```python
from build123d import *

# Parameters (mm, degrees)
BOSS_EXTRUDE1_DEPTH = 2
BOSS_EXTRUDE2_START = -17.5
SKETCH2_R           = 1.75
BOSS_EXTRUDE2_DEPTH = 35
SKETCH3_R           = 3
CUT_EXTRUDE1_DEPTH  = 6.75
CUT_EXTRUDE2_DEPTH  = 2
BOSS_EXTRUDE4_START = -0.5
BOSS_EXTRUDE4_DEPTH = 3.5
SKETCH6_R           = 1.75
CUT_EXTRUDE3_DEPTH  = 77.941536247
FILLET1_R           = 1
SKETCH7_W           = 9
SKETCH7_H           = 6
CUT_EXTRUDE4_DEPTH  = 2
FILLET2_R           = 3
FILLET3_R           = 3


# Some blends are built 0.0001 mm under size
with BuildPart() as part:
    # Sketch1 → Boss-Extrude1 (new body)
    with BuildSketch(Plane(origin=(0, 0, 0), x_dir=(1, 0, 0), z_dir=(0, 1, 0))):
        with BuildLine():
            Line((-17.5, -42), (17.5, -42))
            ThreePointArc((17.5, -42), (45.5, 0), (17.5, 42))
            Line((17.5, 42), (-17.5, 42))
            ThreePointArc((-17.5, 42), (-45.5, 0), (-17.5, -42))
        make_face()
    extrude(amount=BOSS_EXTRUDE1_DEPTH)

    # Sketch2 → Boss-Extrude2 (add)
    with BuildSketch(Plane(origin=(0, 0, 0), x_dir=(0, 0, -1), z_dir=(1, 0, 0)).offset(BOSS_EXTRUDE2_START)):
        with BuildLine():
            Line((-42, 0), (-42.171572875, 0))
            ThreePointArc((-42.171572875, 0), (-48, 1), (-42.171572875, 2))
            Line((-42.171572875, 2), (-42, 2))
            Line((-42, 2), (-42, 1))
            Line((-42, 1), (-42, 0))
        make_face()
        with Locations((-45, 1)):
            Circle(SKETCH2_R, mode=Mode.SUBTRACT)
    extrude(amount=BOSS_EXTRUDE2_DEPTH)

    # Sketch3 → Cut-Extrude1 (cut)
    with BuildSketch(Plane(origin=(3.5, 0, 0), x_dir=(0, 0, -1), z_dir=(1, 0, 0))):
        with Locations((-45, 1)):
            Circle(SKETCH3_R)
    cut_extrude1 = extrude(amount=CUT_EXTRUDE1_DEPTH, mode=Mode.SUBTRACT)

    # Mirror1: Cut-Extrude1 across plane
    add(cut_extrude1.mirror(Plane(origin=(0, 0, 0), x_dir=(0, 0, 1), z_dir=(1, 0, 0))), mode=Mode.SUBTRACT)

    # Sketch4 → Cut-Extrude2 (cut)
    with BuildSketch(Plane(origin=(0, 2, 0), x_dir=(1, 0, 0), z_dir=(0, 1, 0))):
        Polygon((0.75, 42), (21.25, 42), (21.25, 32.75), (0.75, 32.75), (0.75, 35), (-17.5, 35), (-17.5, 42), align=None)
    extrude(amount=-CUT_EXTRUDE2_DEPTH, mode=Mode.SUBTRACT)

    # Sketch5 → Boss-Extrude4 (add)
    with BuildSketch(Plane(origin=(-17.5, 0, 0), x_dir=(0, 0, -1), z_dir=(1, 0, 0)).offset(BOSS_EXTRUDE4_START)):
        with BuildLine():
            Line((35, 1), (35, 2))
            Line((35, 2), (38.171572875, 2))
            ThreePointArc((38.171572875, 2), (44, 1), (38.171572875, 0))
            Line((38.171572875, 0), (35, 0))
            Line((35, 0), (35, 1))
        make_face()
    extrude(amount=BOSS_EXTRUDE4_DEPTH)

    # Sketch6 → Cut-Extrude3 (cut, through all)
    with BuildSketch(Plane(origin=(-14.5, 0, 0), x_dir=(0, 0, -1), z_dir=(1, 0, 0))):
        with Locations((41, 1)):
            Circle(SKETCH6_R)
    extrude(amount=-CUT_EXTRUDE3_DEPTH, mode=Mode.SUBTRACT)

    # Fillet1
    fillet1_edges = [part.edges().sort_by_distance(p)[0] for p in [
        (-20.235557777, 0, -39.563859338),
        (-20.235557777, 2, -39.563859338),
    ]]
    fillet(fillet1_edges, radius=FILLET1_R - 0.0001)  # a hair under: the kernel refuses the full size

    # Sketch7 → Cut-Extrude4 (cut)
    with BuildSketch(Plane(origin=(0, 2, 0), x_dir=(1, 0, 0), z_dir=(0, 1, 0))):
        with Locations((24.75, 38)):
            Rectangle(SKETCH7_W, SKETCH7_H)
    extrude(amount=-CUT_EXTRUDE4_DEPTH, mode=Mode.SUBTRACT)

    # Fillet2
    # the kernel refuses this fillet: 3 mm, written as the material it adds along each edge
    with BuildSketch(Plane(origin=(-14.5, 0, -35), x_dir=(0, 0, -1), z_dir=(0, 1, 0))) as fillet2_piece_1:
        with BuildLine():
            CenterArc((FILLET2_R, -FILLET2_R), FILLET2_R, 90, 90)
            Line((0, -FILLET2_R), (0, 0))
            Line((0, 0), (FILLET2_R, 0))
        make_face()
    extrude(amount=2)
    # the kernel refuses this fillet: 3 mm, written as the material it takes off along each edge
    with BuildSketch(Plane(origin=(29.07318352, 4.856917414, -35), x_dir=(-1, 0, 0), z_dir=(0, -1, 0))) as fillet2_2_piece_1:
        with BuildLine():
            CenterArc((1.104450978, -3), FILLET2_R, 90, 41.15420196)
            ThreePointArc((-0.869812495, -0.741176471), (-0.43723324, -0.367857378), (0, 0))
            Line((0, 0), (1.104450978, 0))
        make_face()
    extrude(amount=7.713834827, mode=Mode.SUBTRACT)
    with BuildSketch(Plane(origin=(21.25, -7.261843774, -35), x_dir=(0, 0, 1), z_dir=(0, 1, 0))) as fillet2_2_piece_2:
        with BuildLine():
            CenterArc((3, 2.90473751), FILLET2_R, 180, 75.522487814)
            Line((0, 2.90473751), (0, 0))
            Line((0, 0), (2.25, 0))
        make_face()
    extrude(amount=16.523687548, mode=Mode.SUBTRACT)
    with BuildSketch(Plane(origin=(0.75, 9.261843774, -35), x_dir=(-1, 0, 0), z_dir=(0, -1, 0))) as fillet2_2_piece_3:
        with BuildLine():
            CenterArc((2.90473751, -3), FILLET2_R, 90, 75.522487814)
            Line((0, -2.25), (0, 0))
            Line((0, 0), (2.90473751, 0))
        make_face()
    extrude(amount=16.523687548, mode=Mode.SUBTRACT)

    # Fillet3
    fillet3_edges = [part.edges().sort_by_distance(p)[0] for p in [
        (21.25, 1, -32.75),
        (0.75, 1, -32.75),
    ]]
    fillet(fillet3_edges, radius=FILLET3_R)


solid = part.part
```
Geometry: final body of the model. Coordinates: model frame, mm. A direction names the side the tool comes from. Round coordinates to 2 decimals unless told otherwise and drop trailing zeros. Order: outer loops, then holes, each group sorted by start corner. A loop starts at its lowest first (then second) coordinate and runs counter-clockwise, first axis right, second up. Notation, with made-up numbers: (84, 63.25) -> (108, 63.25) arc R9 ccw to (108, 74.25) -> close; hole circle Ø5 at (35.25, 21). An arc over 180 degrees is marked (long way). Use CSV: the item, a comma, the result in double quotes. Start each with the question number.
1) Draft query along Y for faces 5 (the face through (0, 1, 48)), 6 (the face through (-13.64, 0.99, -35.9)), 7 (the face through (7, 1, 42)). Return one class per face: +Y half, -Y half, draft (parallel to the pull), parting line (faces both ways), or undercut.
2) Set-up query: faces 1 (the face through (-7, 1, -35)), 2 (the face through (11, 1, -32.75)), 3 (the face through (17.5, 1, 47)), 4 (the face through (-7, 1, 42)). Return all of +Z, -Z, +X, -X, +Y, -Y with unobstructed straight access to the full face (end or side cutting, diameter ignored); none if empty.
3) Section D-D (z = -2). Return the cut outline in (x, y), and give its area (3 significant figures).
4) First-contact query: pin 1 Ø3 at (x, z) = (-10.5, 13.5) entering from +Y; pin 2 Ø3 at (y, z) = (1.5, 44) entering from +X; pin 3 Ø2 at (x, y) = (-7, 1) entering from -Z; pin 4 Ø1.8 at (y, z) = (1.5, 45) entering from +X. Flat tips, straight axial feed; report the tip coordinate or a pass-through.
5) Section C-C (x = -34.5). Return the cut outline in (y, z).
6) Material intervals for line 1 along Y through (x, z) = (13, 45); line 2 along Z through (x, y) = (12.25, 1); line 3 along Y through (x, z) = (39, 5), sorted ascending. Write a range as from..to.
7) Section B-B (z = 45). Return the cut outline in (x, y), and give its area (4 significant figures).
8) Section A-A (z = -41). Return the cut outline in (x, y), and give its area (3 significant figures).
Returned:
1,face 5,"parting line"
1,face 6,"draft"
1,face 7,"undercut"
2,face 1,"-Z, +X, +Y, -Y"
2,face 2,"-Z, +Y, -Y"
2,face 3,"+Z, +X, +Y, -Y"
2,face 4,"+Z"
3,outline,"(-45.46, 0) -> (45.46, 0) -> (45.46, 2) -> (-45.46, 2) -> close"
3,area,"182 mm²"
4,pin 1,"stops at y = 2"
4,pin 2,"stops at x = 17.5"
4,pin 3,"stops at z = -35"
4,pin 4,"passes through"
5,outline,"(0, -29.66) -> (2, -29.66) -> (2, 29.66) -> (0, 29.66) -> close"
6,line 1,"y = -2..-0.75, 2.75..4"
6,line 2,"z = -32.75..43.25, 46.75..48"
6,line 3,"y = 0..2"
7,outline,"(-17.5, -2) -> (-10.25, -2) -> (-10.25, -0.75) -> (-17.5, -0.75) -> close; (-17.5, 2.75) -> (-10.25, 2.75) -> (-10.25, 4) -> (-17.5, 4) -> close; (-3.5, -2) -> (3.5, -2) -> (3.5, -0.75) -> (-3.5, -0.75) -> close; (-3.5, 2.75) -> (3.5, 2.75) -> (3.5, 4) -> (-3.5, 4) -> close; (10.25, -2) -> (17.5, -2) -> (17.5, -0.75) -> (10.25, -0.75) -> close; (10.25, 2.75) -> (17.5, 2.75) -> (17.5, 4) -> (10.25, 4) -> close"
7,area,"53.75 mm²"
8,outline,"(-18, -2) -> (-14.5, -2) -> (-14.5, -0.75) -> (-18, -0.75) -> close; (-18, 2.75) -> (-14.5, 2.75) -> (-14.5, 4) -> (-18, 4) -> close"
8,area,"8.75 mm²"
